Can you work these out from the model? Positions are in its coordinate system, mm. A direction names the side the tool comes from. Round coordinates to 2 decimals unless told otherwise and drop trailing zeros. Loops run counter-clockwise (first coordinate to the right, second up) from the corner with the lowest first, then second, coordinate; pieces in that order, holes last. Notation, with made-up numbers: (-34, 73.25) -> (-5, 73.25) arc R21 ccw to (-5, 106.25) -> close; hole circle Ø4 at (66.5, -26). An arc over 180 degrees is marked (long way). Answer as a JSON object with one key per item and string values.
```python
from build123d import *

# Parameters (mm, degrees)
SKETCH6_R          = 1.65
CUT_EXTRUDE1_DEPTH = 2


with BuildPart() as part:
    # Sketch1 → Revolve1 (revolve)
    with BuildSketch(Plane.XY, mode=Mode.PRIVATE) as revolve1_sk:
        Polygon((-7.95, 12.397619048), (-22.95, 12.397619048), (-22.95, 10.397619048), (-12.95, 10.397619048), (-12.95, -0.302380952), (-7.95, -0.302380952), align=None)
    revolve(revolve1_sk.sketch.rotate(Axis((0, 15.542380952, 0), (0, -1, 0)), 270), axis=Axis((0, 15.542380952, 0), (0, -1, 0)))

    # Sketch5 → M3.5 Clearance Hole1 (revolve, cut)
    with BuildSketch(Plane.ZX.offset(5.047619048)):
        Polygon((0, 0), (0, 15.141678207), (1.95, 13.97), (1.95, 0), align=None)
    revolve(axis=Axis((-6.35, 5.047619048, 0), (1, 0, 0)), mode=Mode.SUBTRACT)

    # Sketch6 → Cut-Extrude1 (cut)
    with BuildSketch(Plane.XZ.offset(-10.397619048)):
        with BuildLine():
            ThreePointArc((1.65, 17.95), (1.166726189, 19.116726189), (0, 19.6))
            Line((0, 19.6), (0, 16.3))
            ThreePointArc((0, 16.3), (1.166726189, 16.783273811), (1.65, 17.95))
        make_face()
        with BuildLine():
            Line((0, 16.3), (0, 19.6))
            ThreePointArc((0, 19.6), (-1.65, 17.95), (0, 16.3))
        make_face()
        with Locations(Location((17.95, 0, 0), (0, 0, 270))):
            Circle(SKETCH6_R)
        with BuildLine():
            ThreePointArc((1.65, -17.95), (1.166726189, -16.783273811), (0, -16.3))
            Line((0, -16.3), (0, -19.6))
            ThreePointArc((0, -19.6), (1.166726189, -19.116726189), (1.65, -17.95))
        make_face()
        with BuildLine():
            Line((0, -19.6), (0, -16.3))
            ThreePointArc((0, -16.3), (-1.65, -17.95), (0, -19.6))
        make_face()
        with Locations(Location((-17.95, 0, 0), (0, 0, 270))):
            Circle(SKETCH6_R)
    extrude(amount=-CUT_EXTRUDE1_DEPTH, mode=Mode.SUBTRACT)


solid = part.part
```
Q1. I want a section at D-D, the plane y = 2. Write out the boundary of the cut face in (x, z), then the cut area to 3 significant figures.
Determined:
{"outline": "circle Ø25.9 at (0, 0); hole circle Ø15.9 at (0, 0)", "area": "328 mm²"}
Q2. I want a section at A-A, the plane z = 0. Write out the boundary of the cut face in (x, y).
Determined:
{"outline": "(-22.95, 10.4) -> (-19.6, 10.4) -> (-19.6, 12.4) -> (-22.95, 12.4) -> close; (-16.3, 10.4) -> (-12.95, 10.4) -> (-12.95, -0.3) -> (-7.95, -0.3) -> (-7.95, 12.4) -> (-16.3, 12.4) -> close; (7.95, -0.3) -> (12.95, -0.3) -> (12.95, 3.1) -> (7.95, 3.1) -> close; (7.95, 7) -> (12.95, 7) -> (12.95, 10.4) -> (16.3, 10.4) -> (16.3, 12.4) -> (7.95, 12.4) -> close; (19.6, 10.4) -> (22.95, 10.4) -> (22.95, 12.4) -> (19.6, 12.4) -> close"}
Q3. I want a section at B-B, the plane x = 3. Write out the boundary of the cut face in (y, z).
Determined:
{"outline": "(-0.3, -12.6) -> (10.4, -12.6) -> (10.4, -22.75) -> (12.4, -22.75) -> (12.4, -7.36) -> (-0.3, -7.36) -> close; (-0.3, 7.36) -> (12.4, 7.36) -> (12.4, 22.75) -> (10.4, 22.75) -> (10.4, 12.6) -> (-0.3, 12.6) -> close"}
Q4. I'm going to push flat-ended pins straight in: pin 1 (5 mm diameter, centred on x = 9, y = 8.5, fed in from +Z); pin 2 (5 mm diameter, centred on x = -6.5, z = 18, fed in from -Y); pin 3 (5 mm diameter, centred on y = 10, z = -16, fed in from +X). Where does each tip first touch, or does it pass through?
Determined:
{"pin 1": "z = 21.73", "pin 2": "y = 10.4", "pin 3": "x = 18.54"}
Q5. On a 3-axis mill with a long thin cutter (end or side, diameter ignored), from which of +Z, -Z, +X, -X, +Y, -Y can I reach the whole of each face in a straight line? I mean faces 4 (the flat face through (10, 10.398, 10)), 5 (the cylindrical face through (-7.882, 6.137, -1.035)), 6 (the cylindrical face through (10.29, 6.95, -0.42)). Say none if no direction works.
Determined:
{"face 4": "-Y", "face 5": "+Y, -Y", "face 6": "+X"}
Q6. If I drill on L1, parallel to X at y = 11.15, z = 0; L2, parallel to Y at x = 11.3, z = 0; L3, parallel to Y at x = -18, z = 9.5, over which ranges is the centre line in solid material (lowest first)? Write a range as [from, to].
Determined:
{"L1": "[-22.95, -19.6], [-16.3, -7.95], [7.95, 16.3], [19.6, 22.95]", "L2": "[-0.3, 3.1], [7, 12.4]", "L3": "[10.4, 12.4]"}
Q7. We'd pull the mould along Z, two halves only. Please class faces 1 (the flat face through (0, 12.398, -10)), 2 (the cylindrical face through (16.34, 11.38, 0.36)), 3 (the cylindrical face through (-6.89, 11.38, 21.89)): pulls with the +Z half, pulls with the -Z half, needs draft (parallel to the pull), parting line crosses it, or undercut.
Determined:
{"face 1": "needs draft", "face 2": "undercut", "face 3": "parting line crosses it"}
Q8. I want a section at C-C, the plane x = 12. Write out the boundary of the cut face in (y, z).
Determined:
{"outline": "(-0.3, -4.87) -> (10.4, -4.87) -> (10.4, -19.56) -> (12.4, -19.56) -> (12.4, 19.56) -> (10.4, 19.56) -> (10.4, 4.87) -> (-0.3, 4.87) -> close; hole circle Ø3.9 at (5.05, 0)"}
